```python
from build123d import *

# Parameters (mm, degrees)
ESQUISSE1_W        = 57
ESQUISSE1_H        = 57
ESQUISSE1_R        = 2.55
BOSS_EXTRU_1_DEPTH = 5
BOSS_EXTRU_2_DEPTH = 108
ESQUISSE3_R        = 19.05
BOSS_EXTRU_3_DEPTH = 1.6
ESQUISSE4_R        = 5
BOSS_EXTRU_4_DEPTH = 4
BOSS_EXTRU_5_DEPTH = 20


with BuildPart() as part:
    # Esquisse1 → Boss.-Extru.1 (new body)
    with BuildSketch(Plane.XY):
        with Locations((-10.354214819, -23.958965641)):
            Rectangle(ESQUISSE1_W, ESQUISSE1_H)
        with Locations((-33.854214819, -0.458965641)):
            Circle(ESQUISSE1_R, mode=Mode.SUBTRACT)
        with Locations((13.145785181, -0.458965641)):
            Circle(ESQUISSE1_R, mode=Mode.SUBTRACT)
        with Locations((13.145785181, -47.458965641)):
            Circle(ESQUISSE1_R, mode=Mode.SUBTRACT)
        with Locations((-33.854214819, -47.458965641)):
            Circle(ESQUISSE1_R, mode=Mode.SUBTRACT)
    extrude(amount=BOSS_EXTRU_1_DEPTH)

    # Esquisse2 → Boss.-Extru.2 (add)
    with BuildSketch(Plane(origin=(0, 0, 0), x_dir=(-1, 0, 0), z_dir=(0, 0, -1))):
        with BuildLine():
            Line((-6.145785181, 4.541034359), (26.854214819, 4.541034359))
            ThreePointArc((26.854214819, 4.541034359), (30.368933444, -3.944247016), (38.854214819, -7.458965641))
            Line((38.854214819, -7.458965641), (38.854214819, -40.458965641))
            ThreePointArc((38.854214819, -40.458965641), (30.368933444, -43.973684267), (26.854214819, -52.458965641))
            Line((26.854214819, -52.458965641), (-6.145785181, -52.458965641))
            ThreePointArc((-6.145785181, -52.458965641), (-9.660503807, -43.973684267), (-18.145785181, -40.458965641))
            Line((-18.145785181, -40.458965641), (-18.145785181, -7.458965641))
            ThreePointArc((-18.145785181, -7.458965641), (-9.660503807, -3.944247016), (-6.145785181, 4.541034359))
        make_face()
    extrude(amount=BOSS_EXTRU_2_DEPTH)

    # Esquisse3 → Boss.-Extru.3 (add)
    with BuildSketch(Plane.XY.offset(5)):
        with Locations((-10.354214819, -23.958965641)):
            Circle(ESQUISSE3_R)
    extrude(amount=BOSS_EXTRU_3_DEPTH)

    # Esquisse4 → Boss.-Extru.4 (add)
    with BuildSketch(Plane.XY.offset(6.6)):
        with Locations((-10.354214819, -23.958965641)):
            Circle(ESQUISSE4_R)
    extrude(amount=BOSS_EXTRU_4_DEPTH)

    # Esquisse5 → Boss.-Extru.5 (add)
    with BuildSketch(Plane.XY.offset(10.6)):
        with BuildLine():
            Line((-12.53366429, -19.458965641), (-8.174765347, -19.458965641))
            ThreePointArc((-8.174765347, -19.458965641), (-10.354214819, -28.958965641), (-12.53366429, -19.458965641))
        make_face()
    extrude(amount=BOSS_EXTRU_5_DEPTH)


solid = part.part
```
Verification items for the finished model (mm, model axes). A direction names the side the tool comes from. Give positions to 0.01 mm unless a question says otherwise; leave off trailing zeros. Loops run counter-clockwise (first coordinate to the right, second up) from the corner with the lowest first, then second, coordinate; pieces in that order, holes last.
1. Section check A-A, the plane z = -68.5. Enter the section's corners in (x, y).
2. Section check B-B, the plane x = -14. Enter the section's corners in (y, z).
3. Section check D-D, the plane x = 2.5. Enter the section's corners in (y, z), then the cut area to 3 significant figures.
4. Thickness scan on line 1 (Y direction, x = 13, z = 4); line 2 (Z direction, x = 14.5, y = -43.5); line 3 (Y direction, x = -10.5, z = 11). Record the ranges inside material, lowest first.
5. Mould release check, pull along X, two halves, no side actions. Record for faces 5 (the flat face through (12, -45, 0)), 6 (the flat face through (-38.854, -24, -52)), 7 (the cylindrical face through (-36.4, -0.3, 2.5)): released by +X, released by -X, zero draft, split by the parting line, or undercut.
6. Go/stop test with flat-tipped pins: pin 1 Ø6.5 at (x, y) = (-33.85, -0.46) entering from +Z; pin 2 Ø1 at (x, z) = (-7.5, 8.5) entering from -Y; pin 3 Ø8 at (x, y) = (-20, -44) entering from +Z. Record where each tip stops, or that it passes through.
7. Set-up check for faces 1 (the cylindrical face through (-30.463, -43.881, -53.244)), 2 (the cylindrical face through (-30.276, -3.85, -53.244)), 3 (the flat face through (-6, -28, 6.6)), 4 (the flat face through (10.7, 1.3, 0)): record each of +Z, -Z, +X, -X, +Y, -Y from which the full face is reachable in a straight line by a thin tool's end or side.
8. Section check C-C, the plane y = -21. Enter the section's corners in (x, z).
Geometry says:
1. outline: (-38.85, -40.46) arc R12 cw to (-26.85, -52.46) - (6.15, -52.46) arc R12 cw to (18.15, -40.46) - (18.15, -7.46) arc R12 cw to (6.15, 4.54) - (-26.85, 4.54) arc R12 cw to (-38.85, -7.46) - close
2. outline: (-52.46, -108) - (4.54, -108) - (4.54, 5) - (-5.26, 5) - (-5.26, 6.6) - (-20.54, 6.6) - (-20.54, 30.6) - (-27.38, 30.6) - (-27.38, 6.6) - (-42.66, 6.6) - (-42.66, 5) - (-52.46, 5) - close
3. outline: (-52.46, -108) - (4.54, -108) - (4.54, 5) - (-9.9, 5) - (-9.9, 6.6) - (-38.02, 6.6) - (-38.02, 5) - (-52.46, 5) - close
3. area: 6,490 mm2
4. line 1: y = -52.46 to -50, -44.91 to -3, 2.09 to 4.54
4. line 2: z = 0 to 5
4. line 3: y = -28.96 to -19.46
5. face 5: zero draft
5. face 6: released by -X
5. face 7: undercut
6. pin 1: stops at z = 5
6. pin 2: stops at y = -28.37
6. pin 3: stops at z = 6.6
7. face 1: -Z, -X, -Y
7. face 2: -Z, -X, +Y
7. face 3: +Z
7. face 4: -Z, +X, +Y
8. outline: (-38.85, -108) - (18.15, -108) - (18.15, 5) - (8.46, 5) - (8.46, 6.6) - (-6.32, 6.6) - (-6.32, 30.6) - (-14.38, 30.6) - (-14.38, 6.6) - (-29.17, 6.6) - (-29.17, 5) - (-38.85, 5) - close
